Can you work these out from the model? Positions are in its coordinate system, mm. A direction names the side the tool comes from. Round coordinates to 2 decimals unless told otherwise and drop trailing zeros. Answer as a JSON object with one key per item and string values. Group by question number.
```python
from build123d import *

# Parameters (mm, degrees)
SKETCH1_W                                   = 27.7
SKETCH1_H                                   = 22
BOSS_EXTRUDE1_DEPTH                         = 22
CUT_EXTRUDE1_DEPTH                          = 38.04443278
CUT_EXTRUDE2_DEPTH                          = 38.04443278
SKETCH4_W                                   = 13.5
SKETCH4_H                                   = 4
CUT_EXTRUDE3_DEPTH                          = 38.04443278
SKETCH5_W                                   = 3.25
SKETCH5_H                                   = 1.8
CUT_EXTRUDE4_DEPTH                          = 38.04443278
CUT_EXTRUDE5_DEPTH                          = 38.04443278
SKETCH7_W                                   = 6
SKETCH7_H                                   = 1.6
CUT_EXTRUDE6_DEPTH                          = 35.056166842
SKETCH8_R                                   = 2.675
CUT_EXTRUDE7_DEPTH                          = 4.5
CUT_EXTRUDE8_DEPTH                          = 3.6
SKETCH10_R                                  = 2
CUT_EXTRUDE9_DEPTH                          = 3
SKETCH15_W                                  = 4
SKETCH15_H                                  = 3
SKETCH15_R                                  = 1.45
BOSS_EXTRUDE4_DEPTH                         = 6.8
SKETCH11_W                                  = 10.5
SKETCH11_H                                  = 7.7
BOSS_EXTRUDE2_DEPTH                         = 4
SKETCH12_R                                  = 3
CUT_EXTRUDE10_DEPTH                         = 3.5
SKETCH13_R                                  = 1.5
REIK_MAHTUU_3_3MM_NIITTI_L_PI_KOSKA_M_DEPTH = 33.905508657
FILLET2_R                                   = 2
FILLET3_R                                   = 1
BOSS_EXTRUDE5_DEPTH                         = 1.15
SKETCH18_W                                  = 1
SKETCH18_H                                  = 1.8
BOSS_EXTRUDE6_DEPTH                         = 4
SKETCH19_W                                  = 8.5
SKETCH19_H                                  = 4
CUT_EXTRUDE12_DEPTH                         = 35.699351643


with BuildPart() as part:
    # Sketch1 → Boss-Extrude1 (new body)
    with BuildSketch(Plane(origin=(0, 0, 0), x_dir=(1, 0, 0), z_dir=(0, 1, 0))):
        Rectangle(SKETCH1_W, SKETCH1_H)
    extrude(amount=BOSS_EXTRUDE1_DEPTH)

    # Sketch2 → Cut-Extrude1 (cut, through all)
    with BuildSketch(Plane(origin=(13.85, 0, 0), x_dir=(0, 0, -1), z_dir=(1, 0, 0))):
        Polygon((-8.4, 22), (-8.4, 21.2), (-11, 14.3), (-11, 22), align=None)
        Polygon((11, 22), (11, 14.3), (8.4, 21.2), (8.4, 22), align=None)
    extrude(amount=-CUT_EXTRUDE1_DEPTH, mode=Mode.SUBTRACT)

    # Sketch3 → Cut-Extrude2 (cut, through all)
    with BuildSketch(Plane(origin=(13.85, 0, 0), x_dir=(0, 0, -1), z_dir=(1, 0, 0))):
        Polygon((-1.55, 22), (1.55, 22), (1.5, 14.700171235), (-1.5, 14.700171235), align=None)
    extrude(amount=-CUT_EXTRUDE2_DEPTH, mode=Mode.SUBTRACT)

    # Sketch4 → Cut-Extrude3 (cut, through all)
    with BuildSketch(Plane(origin=(13.85, 0, 0), x_dir=(0, 0, -1), z_dir=(1, 0, 0))):
        with Locations((0, 2)):
            Rectangle(SKETCH4_W, SKETCH4_H)
    extrude(amount=-CUT_EXTRUDE3_DEPTH, mode=Mode.SUBTRACT)

    # Sketch5 → Cut-Extrude4 (cut, through all)
    with BuildSketch(Plane(origin=(13.85, 0, 0), x_dir=(0, 0, -1), z_dir=(1, 0, 0))):
        with Locations((-8.375, 3.1)):
            Rectangle(SKETCH5_W, SKETCH5_H)
        with Locations((8.375, 3.1)):
            Rectangle(SKETCH5_W, SKETCH5_H)
    extrude(amount=-CUT_EXTRUDE4_DEPTH, mode=Mode.SUBTRACT)

    # Sketch6 → Cut-Extrude5 (cut, through all)
    with BuildSketch(Plane(origin=(13.85, 0, 0), x_dir=(0, 0, -1), z_dir=(1, 0, 0))):
        Polygon((-8.2, 0), (-6.75, 2.2), (-6.75, 0), align=None)
        Polygon((6.75, 0), (8.2, 0), (6.75, 2.2), align=None)
    extrude(amount=-CUT_EXTRUDE5_DEPTH, mode=Mode.SUBTRACT)

    # Sketch7 → Cut-Extrude6 (cut, through all)
    with BuildSketch(Plane.XY.offset(11)):
        with Locations((-7.5, 3.1)):
            Rectangle(SKETCH7_W, SKETCH7_H)
        with Locations((7.5, 3.1)):
            Rectangle(SKETCH7_W, SKETCH7_H)
    extrude(amount=-CUT_EXTRUDE6_DEPTH, mode=Mode.SUBTRACT)

    # Sketch8 → Cut-Extrude7 (cut)
    with BuildSketch(Plane(origin=(0, 22, 0), x_dir=(1, 0, 0), z_dir=(0, 1, 0))):
        with Locations(Location((-9.9, 5, 0), (0, 0, 270))):
            Circle(SKETCH8_R)
        with Locations(Location((-3.3, 5, 0), (0, 0, 270))):
            Circle(SKETCH8_R)
        with Locations(Location((3.3, 5, 0), (0, 0, 270))):
            Circle(SKETCH8_R)
        with Locations(Location((9.9, 5, 0), (0, 0, 270))):
            Circle(SKETCH8_R)
        with Locations(Location((9.9, -5, 0), (0, 0, 270))):
            Circle(SKETCH8_R)
        with Locations(Location((3.3, -5, 0), (0, 0, 270))):
            Circle(SKETCH8_R)
        with Locations(Location((-3.3, -5, 0), (0, 0, 270))):
            Circle(SKETCH8_R)
        with Locations(Location((-9.9, -5, 0), (0, 0, 270))):
            Circle(SKETCH8_R)
    extrude(amount=-CUT_EXTRUDE7_DEPTH, mode=Mode.SUBTRACT)

    # Sketch9 → Cut-Extrude8 (cut)
    with BuildSketch(Plane.XY.offset(11)):
        Polygon((-7.75, 12.7), (-7.5, 11), (-7.5, 6), (-13.5, 6), (-13.5, 11), (-13.25, 12.7), align=None)
        Polygon((-0.75, 12.7), (-0.5, 11), (-0.5, 6), (-6.5, 6), (-6.5, 11), (-6.25, 12.7), align=None)
        Polygon((6.25, 12.7), (6.5, 11), (6.5, 6), (0.5, 6), (0.5, 11), (0.75, 12.7), align=None)
        Polygon((13.25, 12.7), (13.5, 11), (13.5, 6), (7.5, 6), (7.5, 11), (7.75, 12.7), align=None)
    cut_extrude8 = extrude(amount=-CUT_EXTRUDE8_DEPTH, mode=Mode.SUBTRACT)

    # Mirror1: Cut-Extrude8 across plane
    add(cut_extrude8.mirror(Plane.XY), mode=Mode.SUBTRACT)

    # Sketch10 → Cut-Extrude9 (cut)
    with BuildSketch(Plane.XY.offset(7.4)):
        with Locations((-10.5, 8.5)):
            Circle(SKETCH10_R)
        with Locations((-3.5, 8.5)):
            Circle(SKETCH10_R)
        with Locations((3.5, 8.5)):
            Circle(SKETCH10_R)
        with Locations((10.5, 8.5)):
            Circle(SKETCH10_R)
    cut_extrude9 = extrude(amount=-CUT_EXTRUDE9_DEPTH, mode=Mode.SUBTRACT)

    # Mirror2: Cut-Extrude9 across plane
    add(cut_extrude9.mirror(Plane.XY), mode=Mode.SUBTRACT)

    # Sketch15 → Boss-Extrude4 (add)
    # profile 1 of 2: a face of its own
    with BuildSketch(Plane(origin=(0, 14.700171235, 0), x_dir=(1, 0, 0), z_dir=(0, 1, 0))):
        with Locations((-6.5, 0)):
            Rectangle(SKETCH15_W, SKETCH15_H)
        with Locations(Location((-6.5, 0, 0), (0, 0, 270))):
            Circle(SKETCH15_R, mode=Mode.SUBTRACT)
    # profile 2 of 2: a face of its own
    with BuildSketch(Plane(origin=(0, 14.700171235, 0), x_dir=(1, 0, 0), z_dir=(0, 1, 0))):
        with Locations((6.5, 0)):
            Rectangle(SKETCH15_W, SKETCH15_H)
        with Locations(Location((6.5, 0, 0), (0, 0, 270))):
            Circle(SKETCH15_R, mode=Mode.SUBTRACT)
    extrude(amount=BOSS_EXTRUDE4_DEPTH)

    # Sketch11 → Boss-Extrude2 (add)
    with BuildSketch(Plane.XZ.offset(-4)):
        with Locations((17.1, 0)):
            Rectangle(SKETCH11_W, SKETCH11_H)
    extrude(amount=BOSS_EXTRUDE2_DEPTH)

    # Sketch12 → Cut-Extrude10 (cut)
    with BuildSketch(Plane(origin=(0, 4, 0), x_dir=(1, 0, 0), z_dir=(0, 1, 0))):
        with Locations(Location((18.35, 0, 0), (0, 0, 270))):
            Circle(SKETCH12_R)
    extrude(amount=-CUT_EXTRUDE10_DEPTH, mode=Mode.SUBTRACT)

    # Sketch13 → Reikä. Mahtuu 3,3mm niitti läpi, koska materiaali muovia (cut, through all)
    with BuildSketch(Plane(origin=(0, 0.5, 0), x_dir=(1, 0, 0), z_dir=(0, 1, 0))):
        with Locations(Location((18.35, 0, 0), (0, 0, 270))):
            Circle(SKETCH13_R)
    extrude(amount=-REIK_MAHTUU_3_3MM_NIITTI_L_PI_KOSKA_M_DEPTH, mode=Mode.SUBTRACT)

    # Fillet2
    fillet2_edges = [part.edges().sort_by_distance(p)[0] for p in [
        (17.1, 0, -3.85),
        (11.85, 0, 0),
        (17.1, 0, 3.85),
        (22.35, 0, 0),
    ]]
    fillet(fillet2_edges, radius=FILLET2_R)

    # Fillet3
    fillet3_edges = [part.edges().sort_by_distance(p)[0] for p in [
        (22.35, 3, -3.85),
        (22.35, 3, 3.85),
        (21.642097815, 0.473407966, 3.142097815),
        (21.642097815, 0.473407966, -3.142097815),
    ]]
    fillet(fillet3_edges, radius=FILLET3_R)

    # Sketch16 → Boss-Extrude5 (add, symmetric)
    with BuildSketch(Plane.XY):
        Polygon((11.85, 2), (11.85, 4), (9.85, 4), align=None)
    extrude(amount=BOSS_EXTRUDE5_DEPTH, both=True)

    # Sketch18 → Boss-Extrude6 (add)
    with BuildSketch(Plane.XZ.offset(-4)):
        with Locations((2.35, 9.1)):
            Rectangle(SKETCH18_W, SKETCH18_H)
        with Locations((2.35, -9.1)):
            Rectangle(SKETCH18_W, SKETCH18_H)
    extrude(amount=BOSS_EXTRUDE6_DEPTH)

    # Sketch19 → Cut-Extrude12 (cut, through all)
    with BuildSketch(Plane.XY.offset(3.85)):
        with Locations((18.1, 2)):
            Rectangle(SKETCH19_W, SKETCH19_H)
    extrude(amount=-CUT_EXTRUDE12_DEPTH, mode=Mode.SUBTRACT)


solid = part.part
```
1) Which directions (+Z, -Z, +X, -X, +Y, -Y) give clear straight access to the entire face, cutting with the end or side of a thin tool? Please do faces 5 (the face through (6.5, 9, -9)), 6 (the face through (1.85, 3, 9)), 7 (the face through (12.2, 0.87, 0.05)), 8 (the face through (0.5, 8, 9)).
2) We'd pull the mould along Z, two halves only. Please class faces 1 (the face through (10, 17.5, 5)), 2 (the face through (-4, 3, 10)), 3 (the face through (3, 9, 4.4)), 4 (the face through (3, 9, -4.4)): +Z half, -Z half, draft (parallel to the pull), parting line (faces both ways), or undercut.
3) I need wall thicknesses on line 1 along X through (y, z) = (7.5, 8.75); line 2 along X through (y, z) = (20.25, 0); line 3 along X through (y, z) = (19.95, -5) (3 decimals). Which ranges of each line are inside material? Lowest first, please.
4) For pin 1 (1.2 mm diameter, centred on x = 10.5, y = 7.5, fed in from -Z); pin 2 (4.5 mm diameter, centred on x = -4, y = 9, fed in from -Z); pin 3 (3.5 mm diameter, centred on x = -6.5, z = 0, fed in from -Y), each with a flat end and sliding along its axis, tell me the tip position at first contact or that it passes through.
5) If we section it at A-A on y = 20: Count the separate pieces of the cut face and the enclosed holes in it, plus the area to 3 significant figures.
Findings:
{
 "1": {"face 5": "-Z", "face 6": "-X", "face 7": "-X, -Y", "face 8": "+Z"},
 "2": {"face 1": "undercut", "face 2": "undercut", "face 3": "+Z half", "face 4": "-Z half"},
 "3": {"line 1": "x = -13.85 to -13.5, -7.5 to -6.5, -0.5 to 0.5, 6.5 to 7.5, 13.5 to 13.85", "line 2": "x = -8.5 to -7.95, -5.05 to -4.5, 4.5 to 5.05, 7.95 to 8.5", "line 3": "x = -13.85 to -12.575, -7.225 to -5.975, -0.625 to 0.625, 5.975 to 7.225, 12.575 to 13.85"},
 "4": {"pin 1": "stops at z = -4.4", "pin 2": "stops at z = -7.4", "pin 3": "stops at y = 4"},
 "5": {"separate pieces": "4", "enclosed holes": "10", "area": "236 mm^2"}
}
